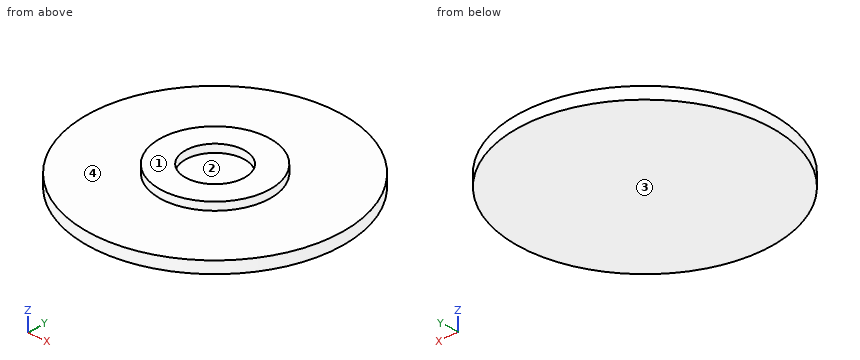
```python
from build123d import *

# Parameters (mm, degrees)
F0_R     = 32.3
F1_DEPTH = 3
F2_R     = 13.95
F3_DEPTH = 5
F4_R     = 7.5
F5_DEPTH = 2


with BuildPart() as f1:
    # F0 (on Top) → F1 (new body)
    with BuildSketch(Plane.XY):
        Circle(F0_R)
    extrude(amount=F1_DEPTH)

    # F2 (on Top) → F3 (join)
    with BuildSketch(Plane.XY):
        Circle(F2_R)
    extrude(amount=F3_DEPTH)

    # F4 (on face) → F5 (cut)
    with BuildSketch(Plane.XY.offset(5)):
        Circle(F4_R)
    extrude(amount=-F5_DEPTH, mode=Mode.SUBTRACT)


solid = f1.part
```
Source: CAD feature listing. Evaluate the final solid. Frame: model axes, mm. Face numbers are marked on the shaded views. A direction names the side the tool comes from. Coordinates: 2 decimals unless noted, no trailing zeros. Write each loop counter-clockwise with the first axis right and the second up, starting at its lowest first coordinate (ties: lowest second). Pieces come first, ordered by that corner, then holes. Notation, with made-up numbers: (18.25, 11) -> (61.25, 11) arc R19 ccw to (61.25, 19) -> close; hole circle Ø2 at (37, 66). An arc over 180 degrees is marked (long way). Return JSON: item names as keys, results as strings. Group by question number.
1) Contact query for a flat-ended pin moving along its axis: P1, Ø10, axis at x = -20.5, y = 24.5, coming from the +Z side. Output: stop coordinate, or through.
2) Section query C-C, the plane z = 4.15. Return loops of the section in (x, y).
3) Set-up query: the marked faces 3 and 4. Return all of +Z, -Z, +X, -X, +Y, -Y with unobstructed straight access to the full face (end or side cutting, diameter ignored); none if empty.
4) Mould query, pull axis X, two halves, no side actions, for the marked faces 1 and 2. Classes: +X half, -X half, draft (parallel to the pull), parting line (faces both ways), or undercut.
5) Ray query, line 1 along Y through (x, z) = (0, 4.25); line 2 along X through (y, z) = (5, 4.3); line 3 along Z through (x, y) = (-13.5, -5). Return the intervals inside material, ascending.
6) Section query A-A, the plane x = 0. Return loops of the section in (y, z).
7) Section query D-D, the plane y = 10. Return loops of the section in (x, z).
From the geometry:
{
 "1": {"P1": "z = 3"},
 "2": {"outline": "circle Ø27.9 at (0, 0); hole circle Ø15 at (0, 0)"},
 "3": {"face 3": "-Z, +X, -X, +Y, -Y", "face 4": "+Z"},
 "4": {"face 1": "draft", "face 2": "undercut"},
 "5": {"line 1": "-13.95 to -7.5, 7.5 to 13.95", "line 2": "-13.02 to -5.59, 5.59 to 13.02", "line 3": "0 to 3"},
 "6": {"outline": "(-32.3, 0) -> (32.3, 0) -> (32.3, 3) -> (13.95, 3) -> (13.95, 5) -> (7.5, 5) -> (7.5, 3) -> (-7.5, 3) -> (-7.5, 5) -> (-13.95, 5) -> (-13.95, 3) -> (-32.3, 3) -> close"},
 "7": {"outline": "(-30.71, 0) -> (30.71, 0) -> (30.71, 3) -> (9.73, 3) -> (9.73, 5) -> (-9.73, 5) -> (-9.73, 3) -> (-30.71, 3) -> close"}
}
